Verification items for the finished model (mm, model axes). A direction names the side the tool comes from. Give positions to 0.01 mm unless a question says otherwise; leave off trailing zeros. Loops run counter-clockwise (first coordinate to the right, second up) from the corner with the lowest first, then second, coordinate; pieces in that order, holes last. Notation, with made-up numbers: (64.5, 19) - (90.5, 19) arc R11 ccw to (90.5, 35) - close; hole circle Ø10 at (52, -5). An arc over 180 degrees is marked (long way). Use one line per item in the form item = value.
```python
from build123d import *

# Parameters (mm, degrees)
F1_DEPTH     = 15
F3_DEPTH     = 8
F4_W         = 7.4894965633
F4_H         = 15
F5_DEPTH     = 8
F6_DEPTH     = 6.7
F7_T4_DEPTH  = 10.9844903399
F7_T10_DEPTH = 10.9844903399
F7_T16_DEPTH = 10.9844903399
F7_T23_DEPTH = 10.9844903399
F7_T29_DEPTH = 10.9844903399
F7_T37_DEPTH = 10.9844903399
F7_T41_DEPTH = 10.9844903399
F7_T48_DEPTH = 10.9844903399
F7_T53_DEPTH = 10.9844903399
F7_T61_DEPTH = 10.9844903399
F7_T66_DEPTH = 10.9844903399
F7_T74_DEPTH = 10.9844903399
F7_T79_DEPTH = 10.9844903399
F7_T86_DEPTH = 10.9844903399
F7_T91_DEPTH = 10.9844903399
F8_R         = 1


# Not quite as in the source:
# - a fillet or chamfer that OpenCascade refuses, or shapes differently, is made with other operations: its cross-section is extruded or revolved along the edge and cut away or added
# - a feature names something its author has since deleted; it is built from what else it names


with BuildPart() as f1:
    # F0 (on Front) → F1 (new body)
    with BuildSketch(Plane.XZ):
        with BuildLine():
            Line((-11.4096143179, 21.3526541356), (-15.244462928, 21.3526541356))
            Line((-15.244462928, 21.3526541356), (-15.244462928, 1.3526541356))
            Line((-15.244462928, 1.3526541356), (10.755537072, 1.3526541356))
            Line((10.755537072, 1.3526541356), (10.755537072, 21.3526541356))
            Line((10.755537072, 21.3526541356), (6.9206884619, 21.3526541356))
            ThreePointArc((6.9206884619, 21.3526541356), (-2.244462928, 7.3526541356), (-11.4096143179, 21.3526541356))
        make_face()
    extrude(amount=F1_DEPTH)

    # F2 (on face) → F3 (cut)
    with BuildSketch(Plane(origin=(0, 0, 1.3526541356), x_dir=(1, 0, 0), z_dir=(0, 0, -1))):
        Polygon((-0.60974224, 9.75), (-3.879183616, 9.75), (-4.8894965633, 6.6405764747), (-2.244462928, 4.7188470506), (0.4005707074, 6.6405764747), align=None)
    extrude(amount=-F3_DEPTH, mode=Mode.SUBTRACT)

    # F4 (on face) → F5 (cut)
    with BuildSketch(Plane(origin=(0, 0, 1.3526541356), x_dir=(1, 0, 0), z_dir=(0, 0, -1))):
        with Locations((-2.2447482816, 7.5)):
            Rectangle(F4_W, F4_H)
        Polygon((0.4005707074, 6.6405764747), (-2.244462928, 4.7188470506), (-4.8894965633, 6.6405764747), (-3.879183616, 9.75), (-0.60974224, 9.75), align=None, mode=Mode.SUBTRACT)
    extrude(amount=-F5_DEPTH, mode=Mode.SUBTRACT)

    # F4 (on face) → F6 (join)
    with BuildSketch(Plane(origin=(0, 0, 1.3526541356), x_dir=(1, 0, 0), z_dir=(0, 0, -1))):
        with Locations((-2.2447482816, 7.5)):
            Rectangle(F4_W, F4_H)
        Polygon((0.4005707074, 6.6405764747), (-2.244462928, 4.7188470506), (-4.8894965633, 6.6405764747), (-3.879183616, 9.75), (-0.60974224, 9.75), align=None, mode=Mode.SUBTRACT)
    extrude(amount=-F6_DEPTH)

    # F7: chamfer of 1.5 on 5 edges, made by hand


with BuildPart() as f7_tool2:
    # F7_s3 → F7_t4 (new body)
    with BuildSketch(Plane(origin=(-0.5921623143, -0.4302311048, 0), x_dir=(0, 0, 1), z_dir=(-0.8090169944, -0.5877852523, 0))):
        Polygon((8.0526541356, -0.9983652494), (6.5526541356, -2.4983652494), (8.0526541356, -2.4983652494), align=None)
    extrude(amount=F7_T4_DEPTH)

    split(bisect_by=Plane(origin=(-3.0193879884, -4.1558310382, 0), x_dir=(0, 0, 1), z_dir=(-0.5877852523, -0.8090169944, 0)), keep=Keep.TOP)

    split(bisect_by=Plane(origin=(-6.3742076477, -2.0711056126, 0), x_dir=(0, 0, 1), z_dir=(0.9510565163, 0.3090169944, 0)), keep=Keep.TOP)


with BuildPart() as f1_1:
    add(f1.part)

    # F7_t1: cut F7_tool2
    add(f7_tool2.part, mode=Mode.SUBTRACT)


with BuildPart() as f7_tool8:
    # F7_s9 → F7_t10 (new body)
    with BuildSketch(Plane(origin=(6.5407615579, -4.7521414374, 0), x_dir=(0, 0, 1), z_dir=(-0.8090169944, 0.5877852523, 0))):
        Polygon((8.0526541356, -3.6368896662), (6.5526541356, -5.1368896662), (8.0526541356, -5.1368896662), align=None)
    extrude(amount=F7_T10_DEPTH)

    split(bisect_by=Plane(origin=(2.3139360678, -0.7518434043, 0), x_dir=(0, 0, 1), z_dir=(-0.9510565163, 0.3090169944, 0)), keep=Keep.TOP)

    split(bisect_by=Plane(origin=(1.4685022485, -2.021219945, 0), x_dir=(0, 0, 1), z_dir=(0.5877852523, -0.8090169944, 0)), keep=Keep.TOP)


with BuildPart() as f1_2:
    add(f1_1.part)

    # F7_t7: cut F7_tool8
    add(f7_tool8.part, mode=Mode.SUBTRACT)


with BuildPart() as f7_tool14:
    # F7_s15 → F7_t16 (new body)
    with BuildSketch(Plane(origin=(-4.1157189289, -12.6668803911, 0), x_dir=(0, 0, 1), z_dir=(0.3090169944, 0.9510565163, 0))):
        Polygon((8.0526541356, 3.9330163646), (6.5526541356, 2.4330163646), (8.0526541356, 2.4330163646), align=None)
    extrude(amount=F7_T16_DEPTH)

    split(bisect_by=Plane.XZ.offset(9.75), keep=Keep.BOTTOM)

    split(bisect_by=Plane(origin=(-3.0193879884, -4.1558310382, 0), x_dir=(0, 0, 1), z_dir=(-0.5877852523, -0.8090169944, 0)), keep=Keep.TOP)

    split(bisect_by=Plane.YZ.offset(1.5), keep=Keep.BOTTOM)


with BuildPart() as f1_3:
    add(f1_2.part)

    # F7_t13: cut F7_tool14
    add(f7_tool14.part, mode=Mode.SUBTRACT)


with BuildPart() as f7_tool21:
    # F7_s22 → F7_t23 (new body)
    with BuildSketch(Plane.YZ.offset(-7.7367080979)):
        Polygon((-9.75, 6.5526541356), (-11.25, 8.0526541356), (-9.75, 8.0526541356), align=None)
    extrude(amount=F7_T23_DEPTH)

    split(bisect_by=Plane(origin=(2.3139360678, -0.7518434043, 0), x_dir=(0, 0, 1), z_dir=(-0.9510565163, 0.3090169944, 0)), keep=Keep.TOP)

    split(bisect_by=Plane(origin=(-6.3742076477, -2.0711056126, 0), x_dir=(0, 0, 1), z_dir=(0.9510565163, 0.3090169944, 0)), keep=Keep.TOP)


with BuildPart() as f1_4:
    add(f1_3.part)

    # F7_t20: cut F7_tool21
    add(f7_tool21.part, mode=Mode.SUBTRACT)


with BuildPart() as f7_tool27:
    # F7_s28 → F7_t29 (new body)
    with BuildSketch(Plane(origin=(0.2926704633, -0.9007470667, 0), x_dir=(0, 0, 1), z_dir=(0.3090169944, -0.9510565163, 0))):
        Polygon((8.0526541356, 8.202238551), (6.5526541356, 6.702238551), (8.0526541356, 6.702238551), align=None)
    extrude(amount=F7_T29_DEPTH)

    split(bisect_by=Plane.XZ.offset(9.75), keep=Keep.BOTTOM)

    split(bisect_by=Plane.YZ.offset(-5.9894965633), keep=Keep.TOP)

    split(bisect_by=Plane(origin=(1.4685022485, -2.021219945, 0), x_dir=(0, 0, 1), z_dir=(0.5877852523, -0.8090169944, 0)), keep=Keep.TOP)


with BuildPart() as f1_5:
    add(f1_4.part)

    # F7_t26: cut F7_tool27
    add(f7_tool27.part, mode=Mode.SUBTRACT)


with BuildPart() as f7_tool35:
    # F7_s36 → F7_t37 (new body)
    with BuildSketch(Plane(origin=(6.5407615579, -4.7521414374, 0), x_dir=(0, 0, 1), z_dir=(-0.8090169944, 0.5877852523, 0))):
        Polygon((8.0526541356, -3.6368896662), (6.5526541356, -5.1368896662), (8.0526541356, -5.1368896662), align=None)
    extrude(amount=F7_T37_DEPTH)

    split(bisect_by=Plane(origin=(1.4685022485, -2.021219945, 0), x_dir=(0, 0, 1), z_dir=(-0.5877852523, 0.8090169944, 0)), keep=Keep.TOP)


with BuildPart() as f7_tool39:
    # F7_s40 → F7_t41 (new body)
    with BuildSketch(Plane(origin=(-0.5921623143, -0.4302311048, 0), x_dir=(0, 0, 1), z_dir=(-0.8090169944, -0.5877852523, 0))):
        Polygon((8.0526541356, -0.9983652494), (6.5526541356, -2.4983652494), (8.0526541356, -2.4983652494), align=None)
    extrude(amount=F7_T41_DEPTH)

    split(bisect_by=Plane(origin=(-3.0193879884, -4.1558310382, 0), x_dir=(0, 0, 1), z_dir=(0.5877852523, 0.8090169944, 0)), keep=Keep.TOP)


with BuildPart() as f7_tool35_1:
    add(f7_tool35.part)

    # F7_t43: intersect F7_tool39
    add(f7_tool39.part, mode=Mode.INTERSECT)


with BuildPart() as f1_6:
    add(f1_5.part)

    # F7_t33: cut F7_tool35
    add(f7_tool35_1.part, mode=Mode.SUBTRACT)


with BuildPart() as f7_tool46:
    # F7_s47 → F7_t48 (new body)
    with BuildSketch(Plane(origin=(-0.5921623143, -0.4302311048, 0), x_dir=(0, 0, 1), z_dir=(-0.8090169944, -0.5877852523, 0))):
        Polygon((8.0526541356, -0.9983652494), (6.5526541356, -2.4983652494), (8.0526541356, -2.4983652494), align=None)
    extrude(amount=F7_T48_DEPTH)

    split(bisect_by=Plane.YZ.offset(-5.9894965633), keep=Keep.TOP)

    split(bisect_by=Plane(origin=(-6.3742076477, -2.0711056126, 0), x_dir=(0, 0, 1), z_dir=(-0.9510565163, -0.3090169944, 0)), keep=Keep.TOP)


with BuildPart() as f7_tool51:
    # F7_s52 → F7_t53 (new body)
    with BuildSketch(Plane(origin=(0.2926704633, -0.9007470667, 0), x_dir=(0, 0, 1), z_dir=(0.3090169944, -0.9510565163, 0))):
        Polygon((8.0526541356, 8.202238551), (6.5526541356, 6.702238551), (8.0526541356, 6.702238551), align=None)
    extrude(amount=F7_T53_DEPTH)

    split(bisect_by=Plane.YZ.offset(-5.9894965633), keep=Keep.TOP)

    split(bisect_by=Plane(origin=(1.4685022485, -2.021219945, 0), x_dir=(0, 0, 1), z_dir=(-0.5877852523, 0.8090169944, 0)), keep=Keep.TOP)


with BuildPart() as f7_tool46_1:
    add(f7_tool46.part)

    # F7_t56: intersect F7_tool51
    add(f7_tool51.part, mode=Mode.INTERSECT)


with BuildPart() as f1_7:
    add(f1_6.part)

    # F7_t44: cut F7_tool46
    add(f7_tool46_1.part, mode=Mode.SUBTRACT)


with BuildPart() as f7_tool59:
    # F7_s60 → F7_t61 (new body)
    with BuildSketch(Plane(origin=(-4.1157189289, -12.6668803911, 0), x_dir=(0, 0, 1), z_dir=(0.3090169944, 0.9510565163, 0))):
        Polygon((8.0526541356, 3.9330163646), (6.5526541356, 2.4330163646), (8.0526541356, 2.4330163646), align=None)
    extrude(amount=F7_T61_DEPTH)

    split(bisect_by=Plane(origin=(-3.0193879884, -4.1558310382, 0), x_dir=(0, 0, 1), z_dir=(0.5877852523, 0.8090169944, 0)), keep=Keep.TOP)

    split(bisect_by=Plane.YZ.offset(1.5), keep=Keep.BOTTOM)


with BuildPart() as f7_tool64:
    # F7_s65 → F7_t66 (new body)
    with BuildSketch(Plane(origin=(6.5407615579, -4.7521414374, 0), x_dir=(0, 0, 1), z_dir=(-0.8090169944, 0.5877852523, 0))):
        Polygon((8.0526541356, -3.6368896662), (6.5526541356, -5.1368896662), (8.0526541356, -5.1368896662), align=None)
    extrude(amount=F7_T66_DEPTH)

    split(bisect_by=Plane(origin=(2.3139360678, -0.7518434043, 0), x_dir=(0, 0, 1), z_dir=(0.9510565163, -0.3090169944, 0)), keep=Keep.TOP)

    split(bisect_by=Plane.YZ.offset(1.5), keep=Keep.BOTTOM)


with BuildPart() as f7_tool59_1:
    add(f7_tool59.part)

    # F7_t69: intersect F7_tool64
    add(f7_tool64.part, mode=Mode.INTERSECT)


with BuildPart() as f1_8:
    add(f1_7.part)

    # F7_t57: cut F7_tool59
    add(f7_tool59_1.part, mode=Mode.SUBTRACT)


with BuildPart() as f7_tool72:
    # F7_s73 → F7_t74 (new body)
    with BuildSketch(Plane.YZ.offset(-7.7367080979)):
        Polygon((-9.75, 6.5526541356), (-11.25, 8.0526541356), (-9.75, 8.0526541356), align=None)
    extrude(amount=F7_T74_DEPTH)

    split(bisect_by=Plane(origin=(2.3139360678, -0.7518434043, 0), x_dir=(0, 0, 1), z_dir=(0.9510565163, -0.3090169944, 0)), keep=Keep.TOP)

    split(bisect_by=Plane.YZ.offset(1.5), keep=Keep.BOTTOM)


with BuildPart() as f7_tool77:
    # F7_s78 → F7_t79 (new body)
    with BuildSketch(Plane(origin=(-4.1157189289, -12.6668803911, 0), x_dir=(0, 0, 1), z_dir=(0.3090169944, 0.9510565163, 0))):
        Polygon((8.0526541356, 3.9330163646), (6.5526541356, 2.4330163646), (8.0526541356, 2.4330163646), align=None)
    extrude(amount=F7_T79_DEPTH)

    split(bisect_by=Plane.XZ.offset(9.75), keep=Keep.TOP)


with BuildPart() as f7_tool72_1:
    add(f7_tool72.part)

    # F7_t81: intersect F7_tool77
    add(f7_tool77.part, mode=Mode.INTERSECT)


with BuildPart() as f1_9:
    add(f1_8.part)

    # F7_t70: cut F7_tool72
    add(f7_tool72_1.part, mode=Mode.SUBTRACT)


with BuildPart() as f7_tool84:
    # F7_s85 → F7_t86 (new body)
    with BuildSketch(Plane.YZ.offset(-7.7367080979)):
        Polygon((-9.75, 6.5526541356), (-11.25, 8.0526541356), (-9.75, 8.0526541356), align=None)
    extrude(amount=F7_T86_DEPTH)

    split(bisect_by=Plane.YZ.offset(-5.9894965633), keep=Keep.TOP)

    split(bisect_by=Plane(origin=(-6.3742076477, -2.0711056126, 0), x_dir=(0, 0, 1), z_dir=(-0.9510565163, -0.3090169944, 0)), keep=Keep.TOP)


with BuildPart() as f7_tool89:
    # F7_s90 → F7_t91 (new body)
    with BuildSketch(Plane(origin=(0.2926704633, -0.9007470667, 0), x_dir=(0, 0, 1), z_dir=(0.3090169944, -0.9510565163, 0))):
        Polygon((8.0526541356, 8.202238551), (6.5526541356, 6.702238551), (8.0526541356, 6.702238551), align=None)
    extrude(amount=F7_T91_DEPTH)

    split(bisect_by=Plane.XZ.offset(9.75), keep=Keep.TOP)


with BuildPart() as f7_tool84_1:
    add(f7_tool84.part)

    # F7_t93: intersect F7_tool89
    add(f7_tool89.part, mode=Mode.INTERSECT)


with BuildPart() as f1_10:
    add(f1_9.part)

    # F7_t82: cut F7_tool84
    add(f7_tool84_1.part, mode=Mode.SUBTRACT)

    # F8
    f8_edges = [f1_10.edges().sort_by_distance(p)[0] for p in [
        (-15.244463, -7.5, 21.352654),
        (10.755537, -7.5, 21.352654),
        (10.755537, -7.5, 1.352654),
        (-15.244463, -7.5, 1.352654),
    ]]
    fillet(f8_edges, radius=F8_R)


solid = f1_10.part
```
1. Depth check by flat-ended pin: pin 1 Ø4 at (x, y) = (5, -8) entering from +Z; pin 2 Ø1 at (x, y) = (4.5, -3.5) entering from +Z; pin 3 Ø1.7 at (x, y) = (-1, -3.5) entering from +Z; pin 4 Ø7.5 at (x, y) = (-1, -12) entering from +Z. Enter the tip coordinate at first touch or a pass-through.
Result set:
pin_1 = 21.35
pin_2 = 10.46
pin_3 = 8.05
pin_4 = 8.69
2. Section check A-A, the plane z = 12.5. Record the cut outline in (x, y).
Result set:
outline = (-15.24, -15) - (-10.99, -15) - (-10.99, 0) - (-15.24, 0) - close; (6.5, -15) - (10.76, -15) - (10.76, 0) - (6.5, 0) - close
3. Draft check along X on faces 1 (the cylindrical face through (-14.94, -7.6, 21.07)), 2 (the flat face through (-0.612, -4.965, 7.313)), 3 (the flat face through (-2, -15, 7)). Enter one of: released by +X, released by -X, zero draft, split by the parting line, or undercut.
Result set:
face_1 = released by -X
face_2 = undercut
face_3 = zero draft
4. Scan lines: probe 1 along Y at (x, z) = (-2, 4.25); probe 2 along X at (y, z) = (-8.75, 3.25); probe 3 along X at (y, z) = (-10, 8.75). Record each from-to range of solid material in increasing order.
Result set:
probe_1 = -15 to -9.75, -4.9 to 0
probe_2 = -15.24 to -4.2, -0.28 to 10.76
probe_3 = -15.24 to -7.34, 2.85 to 10.76
5. Tool access check on faces 4 (the flat face through (-4.391, -8.174, 3.916)), 5 (the flat face through (-2, -2, 8.053)), 6 (the cylindrical face through (-11.46, -7.4, 13.47)), 7 (the flat face through (8, -7, 21.353)), 8 (the flat face through (-5.055, -8.592, 7.313)). Record the directions out of +Z, -Z, +X, -X, +Y, -Y that give a thin tool (end or side, any length) a straight path to the whole face; none if there is none.
Result set:
face_4 = +Z, -Z
face_5 = +Z, +Y, -Y
face_6 = +Y, -Y
face_7 = +Z, +X, -X, +Y, -Y
face_8 = +Z
6. Section check B-B, the plane z = 6.25. Record the cut outline in (x, y), then the cut area to 3 significant figures.
Result set:
outline = (-15.24, -15) - (10.76, -15) - (10.76, 0) - (-15.24, 0) - close; hole (-4.89, -6.64) - (-3.88, -9.75) - (-0.61, -9.75) - (0.4, -6.64) - (-2.24, -4.72) - close
area = 372 mm²
